Part model, mm, in its own coordinate system. Coordinates: 2 decimals unless noted, no trailing zeros. Order: outer loops, then holes, each group sorted by start corner. A loop starts at its lowest first (then second) coordinate and runs counter-clockwise, first axis right, second up.
```python
from build123d import *

# Parameters (mm, degrees)
F0_R          = 12.7
F1_DEPTH      = 254
F3_DEPTH      = 25.4
F3_DEPTH_BACK = 25.4
F5_DEPTH      = 25.4
F5_DEPTH_BACK = 25.4


with BuildPart() as f1:
    # F0 (on Top) → F1 (new body)
    with BuildSketch(Plane.XY):
        Circle(F0_R)
    extrude(amount=F1_DEPTH)

    # F2 (on Front) → F3 (cut, two sides)
    with BuildSketch(Plane.XZ) as f3_sk:
        with BuildLine():
            ThreePointArc((0, 9.525), (2.2450640303, 10.4549359697), (3.175, 12.7))
            ThreePointArc((3.175, 12.7), (-2.2450640303, 14.9450640303), (0, 9.525))
        make_face()
    extrude(amount=-F3_DEPTH, mode=Mode.SUBTRACT)
    extrude(f3_sk.sketch, amount=F3_DEPTH_BACK, mode=Mode.SUBTRACT)

    # F4 (on Front) → F5 (cut, two sides)
    with BuildSketch(Plane.XZ) as f5_sk:
        with BuildLine():
            ThreePointArc((0, 238.125), (2.2450640303, 239.0549359697), (3.175, 241.3))
            ThreePointArc((3.175, 241.3), (-2.2450640303, 243.5450640303), (0, 238.125))
        make_face()
    extrude(amount=-F5_DEPTH, mode=Mode.SUBTRACT)
    extrude(f5_sk.sketch, amount=F5_DEPTH_BACK, mode=Mode.SUBTRACT)


solid = f1.part
```
(1) Slice it at C-C, the plane z = 241.3. Give the cut face in (x, y) (3 decimals).
(2) Drop flat-ended pins along their axis: pin 1 (8 mm diameter, centred on y = 5.5, z = 94, fed in from +X); pin 2 (4 mm diameter, centred on x = -5.5, z = 220, fed in from -Y); pin 3 (1 mm diameter, centred on x = 1.5, z = 200, fed in from -Y); pin 4 (4 mm diameter, centred on x = 0, z = 241.3, fed in from +Y). Give the stop position or say it passes through.
(3) Probe line 1 (Z direction, x = 0.75, y = -0.5); line 2 (X direction, y = -3.25, z = 241.3) (3 decimals); line 3 (Z direction, x = 1.25, y = 0.5). List the from-to ranges inside material, lowest first.
(4) Slice it at D-D, the plane y = -5.25. Give the cut face in (x, z) (3 decimals).
(5) Slice it at A-A, the plane y = 5.5. Give the cut face in (x, z) (3 decimals).
(6) Pull direction Z, two halves, no side cores. Call faces 1 (the face through (0, 0, 254)), 2 (the face through (0, 0, 0)), 3 (the face through (-1.22, -0.18, 9.77)): +Z half, -Z half, draft (parallel to the pull), parting line (faces both ways), or undercut.
(7) Slice it at B-B, the plane z = 89.5. Give the cut face in (x, y), then the cut area to 3 significant figures.
Here are the results:
1. outline: (-3.175, -12.297) - (-3.175, 12.297) arc R12.7 ccw to start; (3.175, -12.297) arc R12.7 ccw to (3.175, 12.297) - close
2. pin 1: stops at x = 12.61
2. pin 2: stops at y = -12.21
2. pin 3: stops at y = -12.66
2. pin 4: passes through
3. line 1: z = 0 to 9.61, 15.79 to 238.21, 244.39 to 254
3. line 2: x = -12.277 to -3.175, 3.175 to 12.277
3. line 3: z = 0 to 9.78, 15.62 to 238.38, 244.22 to 254
4. outline: (-11.564, 0) - (11.564, 0) - (11.564, 254) - (-11.564, 254) - close; hole circle Ø6.35 at (0, 12.7); hole circle Ø6.35 at (0, 241.3)
5. outline: (-11.447, 0) - (11.447, 0) - (11.447, 254) - (-11.447, 254) - close; hole circle Ø6.35 at (0, 12.7); hole circle Ø6.35 at (0, 241.3)
6. face 1: +Z half
6. face 2: -Z half
6. face 3: undercut
7. outline: circle Ø25.4 at (0, 0)
7. area: 507 mm2
